Autodesk Inventor part; units mm, degrees
ref_plane "YZ Plane" through (0, 0, 0) normal (1, 0, 0) x (0, 1, 0)
ref_plane "XZ Plane" through (0, 0, 0) normal (0, 1, 0) x (-1, 0, 0)
ref_plane "XY Plane" through (0, 0, 0) normal (0, 0, 1) x (1, 0, 0)
sketch "スケッチ1" plane through (0, 0, 0) normal (1, 0, 0) x (0, 1, 0)
  line L0 (0, 17.6) -> (0, 0)
  line L1 (0, 0) -> (2.25, 0)
  line L2 (2.25, 0) -> (2.25, 2.6)
  line L3 (2.25, 2.6) -> (1.3, 2.6)
  line L4 (1.3, 2.6) -> (1.3, 17.6)
  line L5 (1.3, 17.6) -> (0, 17.6)
  dimension "d2" = 2.6
  dimension "d10" = 15
  dimension "d11" = 2.6
  dimension "d12" = 4.5
revolve "回転1" add sketch "スケッチ1" angle 360 about axis through (0, 0, 17.6) along (0, 0, -1)
thread "ねじ1"
sketch "スケッチ2" plane through (0, 0, 0) normal (0, 0, -1) x (-1, 0, 0)
  line L0 (0, 1.1547) -> (1, 0.5774)
  line L1 (1, 0.5774) -> (1, -0.5774)
  line L2 (1, -0.5774) -> (0, -1.1547)
  line L3 (0, -1.1547) -> (-1, -0.5774)
  line L4 (-1, -0.5774) -> (-1, 0.5774)
  line L5 (-1, 0.5774) -> (0, 1.1547)
  line L6 (0, 2.25) -> (0, -2.25) construction
  circle A0 centre (0, 0) radius 2.25
  dimension "d7" = 2
extrude "押し出し1" cut sketch "スケッチ2" against normal blind 1.4 contours L0 L1 L2 L3 L4 L5
properties part number "FC-2615EB" material "チタン"
Here's how the part is built. I have some questions about the finished solid (model axes, mm). A direction names the side the tool comes from. Round coordinates to 2 decimals unless told otherwise and drop trailing zeros. Order: outer loops, then holes, each group sorted by start corner. A loop starts at its lowest first (then second) coordinate and runs counter-clockwise, first axis right, second up. Notation, with made-up numbers: M 87.5,65 L 113.5,65 A20 cw 113.5,83 Z; hole C 13,29 d2. An arc over 180 degrees is marked long. Return JSON: item names as keys, results as strings. Group by question number.
1. If we section it at D-D on x = 1.7: List the corners of the cut face in (y, z) for me, then the cut area to 3 significant figures.
2. If we section it at B-B on z = 6: List the corners of the cut face in (x, y) for me, then the cut area to 3 significant figures.
3. Please list where these lines run through material, in increasing order: probe 1 along Z at (x, y) = (0.35, 0.4); probe 2 along X at (y, z) = (0.6, 10); probe 3 along Z at (x, y) = (1.55, 0.55).
4. I'm going to push a flat-ended pin straight in: pin 1 Ø1 at (x, y) = (0, -0.5) entering from -Z. Where does the tip first touch, or does it pass through?
5. If we mould it in two halves opening along X, with no side actions, what happens to faces 1 (the face through (-1.29, -0.17, 10.21)), 2 (the face through (0, 0, 1.4)), 3 (the face through (1, 1, 0))? For each: pulls with the +X half, pulls with the -X half, needs draft (parallel to the pull), parting line crosses it, or undercut.
6. If we section it at A-A on y = 0: List the corners of the cut face in (x, z) for me, then the cut area to 3 significant figures.
7. If we section it at C-C on x = -0.65: List the corners of the cut face in (y, z) for me.
8. On a 3-axis mill with a long thin cutter (end or side, diameter ignored), from which of +Z, -Z, +X, -X, +Y, -Y can I reach the whole of each face in a straight line? I mean faces 4 (the face through (0.51, 0.86, 0.69)), 5 (the face through (-1.5, 0, 2.6)), 6 (the face through (-2.23, -0.29, 1.32)). Say none if no direction works.
Reply:
{
 "1": {"outline": "M -1.47,0 L 1.47,0 L 1.47,2.6 L -1.47,2.6 Z", "area": "7.66 mm^2"},
 "2": {"outline": "C 0,0 d2.6", "area": "5.31 mm^2"},
 "3": {"probe 1": "1.4 to 17.6", "probe 2": "-1.15 to 1.15", "probe 3": "0 to 2.6"},
 "4": {"pin 1": "z = 1.4"},
 "5": {"face 1": "parting line crosses it", "face 2": "undercut", "face 3": "needs draft"},
 "6": {"outline": "M -2.25,0 L -1,0 L -1,1.4 L 1,1.4 L 1,0 L 2.25,0 L 2.25,2.6 L 1.3,2.6 L 1.3,17.6 L -1.3,17.6 L -1.3,2.6 L -2.25,2.6 Z", "area": "47.9 mm^2"},
 "7": {"outline": "M -2.15,0 L -0.78,0 L -0.78,1.4 L 0.78,1.4 L 0.78,0 L 2.15,0 L 2.15,2.6 L 1.13,2.6 L 1.13,17.6 L -1.13,17.6 L -1.13,2.6 L -2.15,2.6 Z"},
 "8": {"face 4": "-Z", "face 5": "+Z", "face 6": "+Z, -Z"}
}
